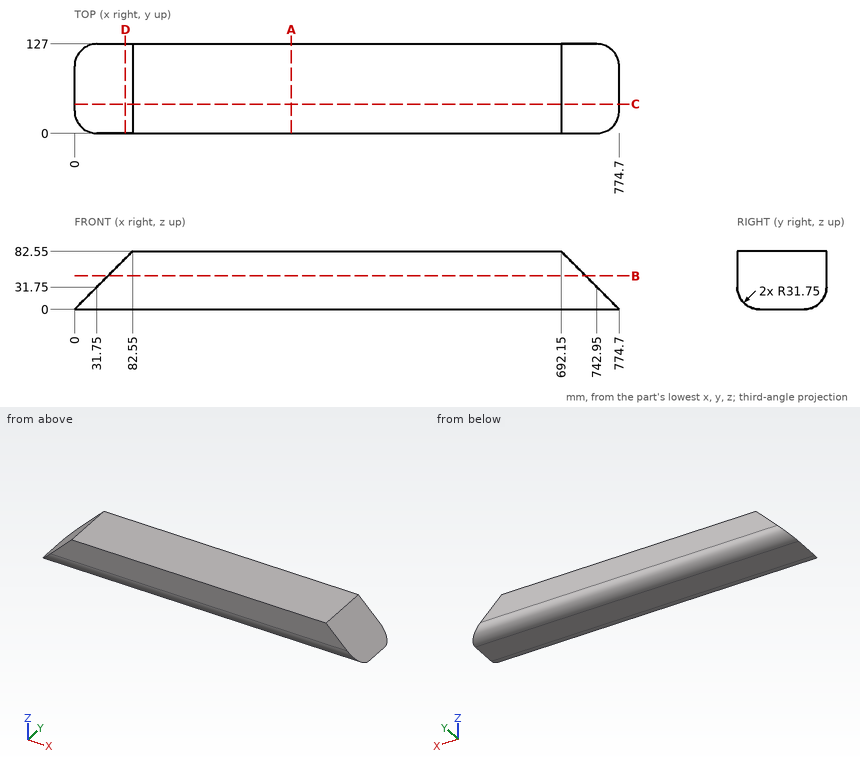
For this review, use the dimensioned drawing (mm, ordinates from the lowest corner) and the shaded views. Give positions to 0.01 mm unless a question says otherwise; leave off trailing zeros. Order: outer loops, then holes, each group sorted by start corner. A loop starts at its lowest first (then second) coordinate and runs counter-clockwise, first axis right, second up. Notation, with made-up numbers: (11, 87.25) - (16, 87.25) arc R31 cw to (16, 111.25) - close; hole circle Ø1 at (39.5, 71). An arc over 180 degrees is marked (long way). Use a Markdown table: item, result. Add a question column.
(1) Add section C-C on y = 41.5. Give the boundary of the cut face in (x, z).
(2) Add section D-D on x = 72.5. Give the boundary of the cut face in (y, z).
(3) Add section B-B on z = 47.5. Give the boundary of the cut face in (x, y).
(4) Wall thickness on probe 1 along Z at (x, y) = (201.5, 97.5); probe 2 along X at (y, z) = (30, 20.5); probe 3 along X at (y, z) = (23, 31.5): over which ranges is each line inside the solid? List them lowest first. Write a range as [from, to].
(5) Clearance check with flat-ended pins moving along their axes: P1, Ø5, axis at x = 405.5, z = 28, coming from the +Y side; P2, Ø1.5, axis at y = 78.5, z = 52.5, coming from the -X side; P3, Ø12, axis at y = 111, z = 20.5, coming from the +X side. State where each tip first meets the part, or that it passes through.
(6) Add section A-A on x = 308.5. Give the boundary of the cut face in (y, z), then the cut area to 3 significant figures.
Report:
| question | item | result |
|---|---|---|
| 1 | outline | (0, 0) - (774.7, 0) - (692.15, 82.55) - (82.55, 82.55) - close |
| 2 | outline | (0, 31.75) arc R31.75 ccw to (31.75, 0) - (95.25, 0) arc R31.75 ccw to (127, 31.75) - (127, 72.5) - (0, 72.5) - close |
| 3 | outline | (47.5, 0) - (727.2, 0) - (727.2, 127) - (47.5, 127) - close |
| 4 | probe 1 | z = [0.08, 82.55] |
| 4 | probe 2 | x = [20.5, 754.2] |
| 4 | probe 3 | x = [31.5, 743.2] |
| 5 | P1 | stops at y = 126.98 |
| 5 | P2 | stops at x = 51.75 |
| 5 | P3 | stops at x = 760.2 |
| 6 | outline | (0, 31.75) arc R31.75 ccw to (31.75, 0) - (95.25, 0) arc R31.75 ccw to (127, 31.75) - (127, 82.55) - (0, 82.55) - close |
| 6 | area | 10,100 mm² |
